```python
from build123d import *

# Parameters (mm, degrees)
SKETCH_2_W           = 80
SKETCH_2_H           = 34
SKETCH_2_R           = 4.05
EXTRUDE_1_DEPTH      = 8
CUT_EXTRUDE_2_DEPTH  = 88.292611371
CUT_EXTRUDE_12_DEPTH = 4.5
SKETCH_20_R          = 6.25
CUT_EXTRUDE_13_DEPTH = 4.5
CUT_EXTRUDE_11_DEPTH = 2
HOLE_WIZARD_M5_1_D   = 4.2
HOLE_WIZARD_M3_1_D   = 2.5
HOLE_WIZARD_M3_2_D   = 2.5
EXTRUDE_2_DEPTH      = 8


with BuildPart() as part:
    # 草图2 → 凸台-拉伸1 (new body)
    with BuildSketch(Plane.XY):
        with Locations((40, 17)):
            Rectangle(SKETCH_2_W, SKETCH_2_H)
        with Locations((7, 8)):
            Circle(SKETCH_2_R, mode=Mode.SUBTRACT)
        with Locations((40, 10)):
            Circle(SKETCH_2_R, mode=Mode.SUBTRACT)
        with Locations((73, 8)):
            Circle(SKETCH_2_R, mode=Mode.SUBTRACT)
    extrude_1 = extrude(amount=EXTRUDE_1_DEPTH)

    # 草图4 → 切除-拉伸2 (cut, through all)
    with BuildSketch(Plane(origin=(80, 0, 0), x_dir=(0, 0, -1), z_dir=(1, 0, 0))):
        Polygon((-1.5, 32.2), (-2.5, 32.2), (-2.5, 34), (0, 34), (0, 28.8), (-1.5, 28.8), align=None)
    cut_extrude_2 = extrude(amount=-CUT_EXTRUDE_2_DEPTH, mode=Mode.SUBTRACT)

    # 草图8 → 切除-拉伸12 (cut)
    with BuildSketch(Plane(origin=(0, 0, 0), x_dir=(-1, 0, 0), z_dir=(0, 0, -1))):
        with BuildLine():
            Line((-30.5, 12.85), (-49.5, 12.85))
            ThreePointArc((-49.5, 12.85), (-52.35, 10), (-49.5, 7.15))
            Line((-49.5, 7.15), (-30.5, 7.15))
            ThreePointArc((-30.5, 7.15), (-27.65, 10), (-30.5, 12.85))
        make_face()
    cut_extrude_12 = extrude(amount=-CUT_EXTRUDE_12_DEPTH, mode=Mode.SUBTRACT)

    # 草图20 → 切除-拉伸13 (cut)
    with BuildSketch(Plane(origin=(0, 0, 0), x_dir=(-1, 0, 0), z_dir=(0, 0, -1))):
        with Locations((-40, 10)):
            Circle(SKETCH_20_R)
    cut_extrude_13 = extrude(amount=-CUT_EXTRUDE_13_DEPTH, mode=Mode.SUBTRACT)

    # 草图19 → 切除-拉伸11 (cut)
    with BuildSketch(Plane(origin=(0, 0, 2.5), x_dir=(-1, 0, 0), z_dir=(0, 0, -1))):
        with BuildLine():
            Line((-25, 34), (-55.247938178, 34))
            Line((-55.247938178, 34), (-55.247938178, 33.2))
            ThreePointArc((-55.247938178, 33.2), (-54.747938178, 32.7), (-54.247938178, 33.2))
            Line((-54.247938178, 33.2), (-26, 33.2))
            ThreePointArc((-26, 33.2), (-25.5, 32.7), (-25, 33.2))
            Line((-25, 33.2), (-25, 34))
        make_face()
    cut_extrude_11 = extrude(amount=-CUT_EXTRUDE_11_DEPTH, mode=Mode.SUBTRACT)

    # M5 螺纹孔1 (through all)
    with Locations(Plane(origin=(57, 8, 8), x_dir=(1, 0, 0), z_dir=(0, 0, 1))):
        with Locations((0, 0), (-34, 0)):
            hole_wizard_m5_1 = Hole(HOLE_WIZARD_M5_1_D / 2)

    # M3 螺纹孔1 (through all)
    with Locations(Plane(origin=(48, 10, 8), x_dir=(1, 0, 0), z_dir=(0, 0, 1))):
        with Locations((0, 0), (-16, 0)):
            hole_wizard_m3_1 = Hole(HOLE_WIZARD_M3_1_D / 2)

    # M3 螺纹孔2 (through all)
    with Locations(Plane(origin=(60, 25, 0), x_dir=(-1, 0, 0), z_dir=(0, 0, -1))):
        with Locations((0, 0), (40, 0)):
            hole_wizard_m3_2 = Hole(HOLE_WIZARD_M3_2_D / 2)

    # 草图22 → 凸台-拉伸2 (add)
    with BuildSketch(Plane.XY.offset(8)):
        with BuildLine():
            Line((0.5, -4), (5.5, -4))
            ThreePointArc((5.5, -4), (3.5, -2), (5.5, 0))
            Line((5.5, 0), (0.5, 0))
            ThreePointArc((0.5, 0), (2.5, -2), (0.5, -4))
        make_face()
        with BuildLine():
            Line((79.5, 0), (74.5, 0))
            ThreePointArc((74.5, 0), (76.5, -2), (74.5, -4))
            Line((74.5, -4), (79.5, -4))
            ThreePointArc((79.5, -4), (77.5, -2), (79.5, 0))
        make_face()
    extrude(amount=-EXTRUDE_2_DEPTH)

    # 镜向2: 凸台-拉伸1, 切除-拉伸2, 切除-拉伸12, 切除-拉伸13, 切除-拉伸11, M5 螺纹孔1, M3 螺纹孔1, M3 螺纹孔2 across plane
    add(extrude_1.mirror(Plane(origin=(0, -2, 0), x_dir=(0, 0, 1), z_dir=(0, -1, 0))))
    add(cut_extrude_2.mirror(Plane(origin=(0, -2, 0), x_dir=(0, 0, 1), z_dir=(0, -1, 0))), mode=Mode.SUBTRACT)
    add(cut_extrude_12.mirror(Plane(origin=(0, -2, 0), x_dir=(0, 0, 1), z_dir=(0, -1, 0))), mode=Mode.SUBTRACT)
    add(cut_extrude_13.mirror(Plane(origin=(0, -2, 0), x_dir=(0, 0, 1), z_dir=(0, -1, 0))), mode=Mode.SUBTRACT)
    add(cut_extrude_11.mirror(Plane(origin=(0, -2, 0), x_dir=(0, 0, 1), z_dir=(0, -1, 0))), mode=Mode.SUBTRACT)
    add(hole_wizard_m5_1.mirror(Plane(origin=(0, -2, 0), x_dir=(0, 0, 1), z_dir=(0, -1, 0))), mode=Mode.SUBTRACT)
    add(hole_wizard_m3_1.mirror(Plane(origin=(0, -2, 0), x_dir=(0, 0, 1), z_dir=(0, -1, 0))), mode=Mode.SUBTRACT)
    add(hole_wizard_m3_2.mirror(Plane(origin=(0, -2, 0), x_dir=(0, 0, 1), z_dir=(0, -1, 0))), mode=Mode.SUBTRACT)


solid = part.part
```
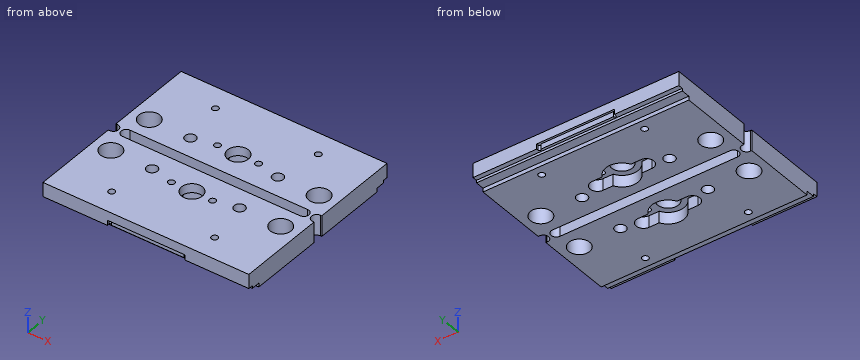
CAD build for the part. Positions are in the model's coordinates, mm. Give positions to 0.01 mm unless a question says otherwise; leave off trailing zeros. Write each loop counter-clockwise with the first axis right and the second up, starting at its lowest first coordinate (ties: lowest second). Pieces come first, ordered by that corner, then holes. Notation, with made-up numbers: M 6.25,34 L 31.25,34 A24 cw 31.25,73 Z; hole C 33,27 d4. An arc over 180 degrees is marked long. Return JSON: item names as keys, results as strings. Group by question number.
(1) Band-saw the part on A-A (x = 63). Give the cut face in (y, z), and give its area (3 significant figures).
(2) Band-saw the part on B-B (z = 6). State how many separate pieces and enclosed holes the cut face has, and give its area (3 significant figures).
(3) Flat gauge pins, fed straight in: pin 1 Ø1.6 at (x, z) = (47, 0.5) entering from -Y; pin 2 Ø6 at (x, y) = (71, 0.5) entering from -Z; pin 3 Ø1 at (x, y) = (46, 31) entering from -Z; pin 4 Ø0.6 at (x, z) = (43.5, 3.5) entering from -Y. Where does each tip first touch, or does it go through?
(4) Band-saw the part on C-C (x = 23). Give the cut face in (y, z).
(5) Band-saw the part on D-D (x = 7). Give the cut face in (y, z), and give its area (3 significant figures).
(6) Drill centre lines: L1, parallel to Y at x = 20, z = 6.25; L2, parallel to Y at x = 32, z = 7.3; L3, parallel to X at y = -30, z = 5. Where is each one in solid material? Low to high. Write a range as [from, to].
Entries:
{
 "1": {"outline": "M -38,2.5 L -36.2,2.5 L -36.2,1.5 L -32.8,1.5 L -32.8,0 L -4,0 L -4,8 L -38,8 Z; M 0,0 L 28.8,0 L 28.8,1.5 L 32.2,1.5 L 32.2,2.5 L 34,2.5 L 34,8 L 0,8 Z", "area": "525 mm^2"},
 "2": {"separate pieces": "1", "enclosed holes": "19", "area": "5,050 mm^2"},
 "3": {"pin 1": "stops at y = -32.8", "pin 2": "stops at z = 0", "pin 3": "stops at z = 1.5", "pin 4": "stops at y = -37.2"},
 "4": {"outline": "M -38,2.5 L -36.2,2.5 L -36.2,1.5 L -32.8,1.5 L -32.8,0 L -14.1,0 L -14.1,8 L -38,8 Z; M -9.9,0 L -4,0 L -4,8 L -9.9,8 Z; M 0,0 L 5.9,0 L 5.9,8 L 0,8 Z; M 10.1,0 L 28.8,0 L 28.8,1.5 L 32.2,1.5 L 32.2,2.5 L 34,2.5 L 34,8 L 10.1,8 Z"},
 "5": {"outline": "M -38,2.5 L -36.2,2.5 L -36.2,1.5 L -32.8,1.5 L -32.8,0 L -16.05,0 L -16.05,8 L -38,8 Z; M -7.95,0 L -4,0 L -4,8 L -7.95,8 Z; M 0,0 L 3.95,0 L 3.95,8 L 0,8 Z; M 12.05,0 L 28.8,0 L 28.8,1.5 L 32.2,1.5 L 32.2,2.5 L 34,2.5 L 34,8 L 12.05,8 Z", "area": "395 mm^2"},
 "6": {"L1": "y = [-38, -30.25], [-27.75, -4], [0, 23.75], [26.25, 34]", "L2": "y = [-38, -15.25], [-12.75, -4], [0, 8.75], [11.25, 34]", "L3": "x = [0, 19.25], [20.75, 59.25], [60.75, 80]"}
}
